The listing builds one solid part. Answer for the finished solid, in the listing's coordinates (mm). Round coordinates to 2 decimals unless told otherwise and drop trailing zeros. Write each loop counter-clockwise with the first axis right and the second up, starting at its lowest first coordinate (ties: lowest second). Pieces come first, ordered by that corner, then holes.
Item 1: Find section B-B on z = 33.6. Give the vertices of the cut face in (x, y).
Item 2: Find section A-A on x = 10.5. Give the vertices of the cut face in (y, z).
Item 3: This flat-tipped pin is pushed along its axis until it touches: pin 1 (4 mm diameter, centred on x = 10.5, z = 33.6, fed in from -Y). Where does it stop, or does it pass through?
Item 4: Find the intervals of material crossed by probe 1 along X at (y, z) = (0.5, -33.6), in increasing order.
Item 5: For a pull along Z with two mould halves and no side action, classify faces 1 (the face through (43.9, 0.51, 36.03)), 2 (the face through (10.966, 0.493, -35.078)), 3 (the face through (-43.93, 0.51, -36)) as +Z half, -Z half, draft (parallel to the pull), parting line (faces both ways), or undercut.
```python
from build123d import *

# Parameters (mm, degrees)
SKETCH_1_W          = 89
SKETCH_1_H          = 73.2
EXTRUDE_1_DEPTH     = 1
SKETCH_2_R          = 1.55
CUT_EXTRUDE_1_DEPTH = 10
FILLET_1_R          = 2


with BuildPart() as part:
    # 草图1 → 凸台-拉伸1 (new body)
    with BuildSketch(Plane(origin=(0, 0, 0), x_dir=(1, 0, 0), z_dir=(0, 1, 0))):
        Rectangle(SKETCH_1_W, SKETCH_1_H)
    extrude(amount=EXTRUDE_1_DEPTH)

    # 草图2 → 切除-拉伸1 (cut)
    with BuildSketch(Plane.XZ):
        with Locations(Location((10.5, 33.6, 0), (0, 0, 270))):
            Circle(SKETCH_2_R)
        with Locations(Location((-9.5, 33.6, 0), (0, 0, 270))):
            Circle(SKETCH_2_R)
        with Locations(Location((-9.5, -33.6, 0), (0, 0, 270))):
            Circle(SKETCH_2_R)
        with Locations(Location((10.5, -33.6, 0), (0, 0, 270))):
            Circle(SKETCH_2_R)
    extrude(amount=-CUT_EXTRUDE_1_DEPTH, mode=Mode.SUBTRACT)

    # 圆角1
    fillet_1_edges = [part.edges().sort_by_distance(p)[0] for p in [
        (44.5, 0.5, 36.6),
        (-44.5, 0.5, 36.6),
        (-44.5, 0.5, -36.6),
        (44.5, 0.5, -36.6),
    ]]
    fillet(fillet_1_edges, radius=FILLET_1_R)


solid = part.part
```
Check values:
1. outline: (-44.5, 0) - (-11.05, 0) - (-11.05, 1) - (-44.5, 1) - close; (-7.95, 0) - (8.95, 0) - (8.95, 1) - (-7.95, 1) - close; (12.05, 0) - (44.5, 0) - (44.5, 1) - (12.05, 1) - close
2. outline: (0, -36.6) - (1, -36.6) - (1, -35.15) - (0, -35.15) - close; (0, -32.05) - (1, -32.05) - (1, 32.05) - (0, 32.05) - close; (0, 35.15) - (1, 35.15) - (1, 36.6) - (0, 36.6) - close
3. pin 1: stops at y = 0
4. probe 1: x = -44.5 to -11.05, -7.95 to 8.95, 12.05 to 44.5
5. face 1: +Z half
5. face 2: undercut
5. face 3: -Z half
